Here's the drawing with two shaded views (mm, measured from the low corner). I have some questions. Give positions to 0.01 mm unless a question says otherwise; leave off trailing zeros. Loops run counter-clockwise (first coordinate to the right, second up) from the corner with the lowest first, then second, coordinate; pieces in that order, holes last. Notation, with made-up numbers: (52.5, -26) - (85.5, -26) arc R14 cw to (85.5, -17) - close; hole circle Ø8 at (9.5, 68). An arc over 180 degrees is marked (long way). Answer as a JSON object with one key per item and string values. Group by question number.
Item 1: Please list where these lines run through material, in increasing order: L1, parallel to Z at x = 1.3, y = 4.23 (1 decimal); L2, parallel to Z at x = 1.8, y = 2.25 (1 decimal); L3, parallel to Y at x = 0.4, z = 4.75 (1 decimal).
Item 2: Thinking about a two-plate mould opening in Z: for the marked faces 1, 2, 3 and 4, which applies, pulls with the +Z half, pulls with the -Z half, needs draft (parallel to the pull), parting line crosses it, or undercut?
Item 3: Suppose I cut it at B-B on x = 1.4. Write out the boundary of the cut face in (y, z) (1 decimal).
Item 4: Suppose I cut it at C-C on y = 4.23. Write out the boundary of the cut face in (x, z) (1 decimal).
Item 5: Suppose I cut it at D-D on y = 8. Write out the boundary of the cut face in (x, z) (1 decimal).
Item 6: Suppose I cut it at A-A on z = 4.5. Write out the boundary of the cut face in (x, y) (1 decimal).
Item 7: Will these pins go through, and if not, where does the flat tip stop? pin 1 (1 mm diameter, centred on x = 0, y = 7, fed in from +Z) (1 decimal); pin 2 (1 mm diameter, centred on x = 0.5, y = 6.5, fed in from -Z).
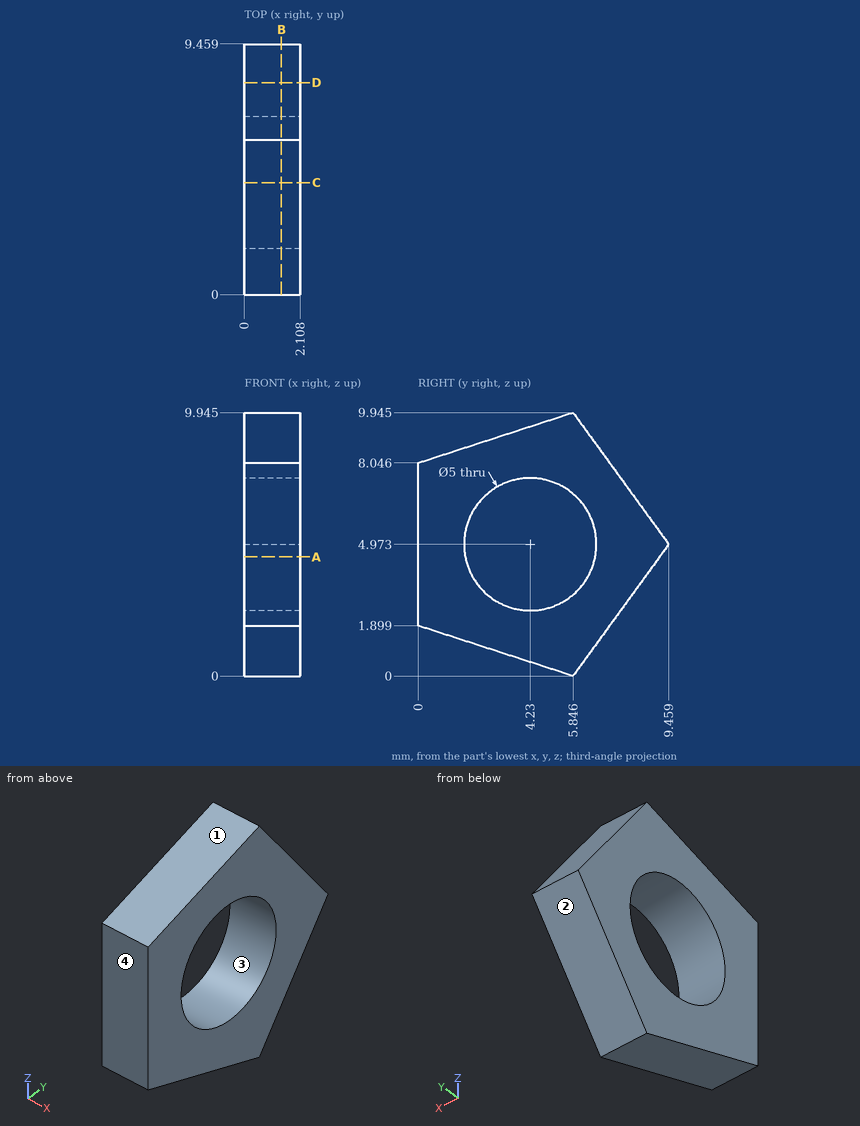
Worked out:
{
 "1": {"L1": "z = 0.5 to 2.5, 7.5 to 9.4", "L2": "z = 1.2 to 3.4, 6.5 to 8.8", "L3": "y = 0 to 1.7, 6.7 to 9.3"},
 "2": {"face 1": "pulls with the +Z half", "face 2": "pulls with the -Z half", "face 3": "undercut", "face 4": "needs draft"},
 "3": {"outline": "(0, 1.9) - (5.8, 0) - (9.5, 5) - (5.8, 9.9) - (0, 8) - close; hole circle Ø5 at (4.2, 5)"},
 "4": {"outline": "(0, 0.5) - (2.1, 0.5) - (2.1, 2.5) - (0, 2.5) - close; (0, 7.5) - (2.1, 7.5) - (2.1, 9.4) - (0, 9.4) - close"},
 "5": {"outline": "(0, 3) - (2.1, 3) - (2.1, 7) - (0, 7) - close"},
 "6": {"outline": "(0, 0) - (2.1, 0) - (2.1, 1.8) - (0, 1.8) - close; (0, 6.7) - (2.1, 6.7) - (2.1, 9.1) - (0, 9.1) - close"},
 "7": {"pin 1": "stops at z = 9", "pin 2": "stops at z = 0.21"}
}
